Can you work these out from the model? Positions are in its coordinate system, mm. Face numbers are marked on the shaded views. A direction names the side the tool comes from. Round coordinates to 2 decimals unless told otherwise and drop trailing zeros. Order: outer loops, then holes, each group sorted by start corner. A loop starts at its lowest first (then second) coordinate and runs counter-clockwise, first axis right, second up. Notation, with made-up numbers: M 42.5,-29 L 87.5,-29 A28 cw 87.5,-9 Z; hole C 17,19.25 d9. An arc over 180 degrees is marked long. Answer as CSV lines item,"result". Start each with the question number.
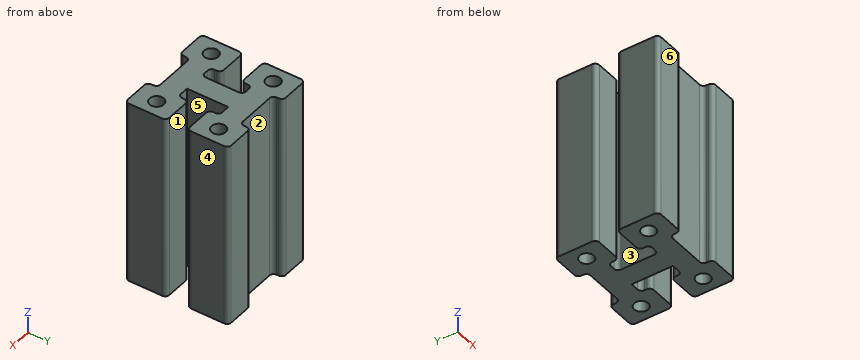
from build123d import *

# Parameters (mm, degrees)
SALIENTE_EXTRUIR1_DEPTH      = 22.4
REDONDEO1_R                  = 1
TALADRO_DE_MARGEN_PARA_M31_D = 3.4


with BuildPart() as part:
    # Croquis1 → Saliente-Extruir1 (new, symmetric)
    with BuildSketch(Plane(origin=(0, 0, 0), x_dir=(0, 1, 0), z_dir=(0, 0, 1))):
        Polygon((-5, 13), (5, 13), (5, 5.5), (2.5, 5.5), (2.5, 2.5), (12.5, 2.5), (12.5, 5.5), (10, 5.5), (10, 13), (20, 13), (20, 5.5), (17.5, 5.5), (17.5, -5.5), (20, -5.5), (20, -13), (10, -13), (10, -5.5), (12.5, -5.5), (12.5, -2.5), (2.5, -2.5), (2.5, -5.5), (5, -5.5), (5, -13), (-5, -13), (-5, -5.5), (-2.5, -5.5), (-2.5, 5.5), (-5, 5.5), align=None)
    extrude(amount=SALIENTE_EXTRUIR1_DEPTH, both=True)

    # Redondeo1
    redondeo1_edges = [part.edges().sort_by_distance(p)[0] for p in [
        (-5.5, -5, 0),
        (-13, -5, 0),
        (-13, 5, 0),
        (-5.5, 5, 0),
        (-5.5, 2.5, 0),
        (-2.5, 2.5, 0),
        (-2.5, 12.5, 0),
        (-5.5, 12.5, 0),
        (-5.5, 10, 0),
        (-13, 10, 0),
        (-13, 20, 0),
        (-5.5, 20, 0),
        (-5.5, 17.5, 0),
        (5.5, 17.5, 0),
        (5.5, 20, 0),
        (13, 20, 0),
        (13, 10, 0),
        (5.5, 10, 0),
        (5.5, 12.5, 0),
        (5.5, 2.5, 0),
        (5.5, 5, 0),
        (13, 5, 0),
        (13, -5, 0),
        (5.5, -5, 0),
        (5.5, -2.5, 0),
        (-5.5, -2.5, 0),
    ]]
    fillet(redondeo1_edges, radius=REDONDEO1_R)

    # Taladro de margen para M31 (through all)
    with Locations(Plane(origin=(0, 0, -22.4), x_dir=(1, 0, 0), z_dir=(0, 0, -1))):
        with Locations((-9.25, -15), (-9.25, 0), (9.25, 0), (9.25, -15)):
            Hole(TALADRO_DE_MARGEN_PARA_M31_D / 2)


solid = part.part
(1) I want a section at B-B on y = 0. Write out the boundary of the cut face in (x, z).
(2) I want a section at C-C on z = 1.5. Count the separate pieces of the cut face and the enclosed holes in it, and give its area (3 significant figures).
(3) I want a section at D-D on y = 15.75. Write out the boundary of the cut face in (x, z), and give its area (3 significant figures).
(4) I'm going to push flat-ended pins straight in: P1, Ø0.8, axis at x = -4, z = 1, coming from the +Y side; P2, Ø2, axis at x = 9.25, y = 15, coming from the -Z side; P3, Ø2, axis at x = 3.5, z = -8.5, coming from the -Y side; P4, Ø10, axis at x = 0, z = -6, coming from the -Y side. Where does each tip first touch, or does it pass through?
(5) If we mould it in two halves opening along X, with no side actions, what happens to the marked faces 4, 5 and 6? For each: +X half, -X half, draft (parallel to the pull), parting line (faces both ways), or undercut.
(6) I want a section at A-A on x = 9.25. Write out the boundary of the cut face in (y, z).
(7) For the marked faces 1, 2 and 3, which set-ups out of +Z, -Z, +X, -X, +Y, -Y let a thin tool reach every point of the face, with its end or its side?
(8) If I drill on line 1 along X through (y, z) = (15, 14); line 2 along Y through (x, z) = (-9.25, 12.5); line 3 along Y through (x, z) = (-11.25, 2), over which ranges is the centre line in solid material (lowest first)?
From the geometry:
1,outline,"M -13,-22.4 L -10.95,-22.4 L -10.95,22.4 L -13,22.4 Z; M -7.55,-22.4 L 7.55,-22.4 L 7.55,22.4 L -7.55,22.4 Z; M 10.95,-22.4 L 13,-22.4 L 13,22.4 L 10.95,22.4 Z"
2,separate pieces,"1"
2,enclosed holes,"4"
2,area,"422 mm²"
3,outline,"M -13,-22.4 L -10.78,-22.4 L -10.78,22.4 L -13,22.4 Z; M -7.72,-22.4 L 7.72,-22.4 L 7.72,22.4 L -7.72,22.4 Z; M 10.78,-22.4 L 13,-22.4 L 13,22.4 L 10.78,22.4 Z"
3,area,"891 mm²"
4,P1,"y = 17.5"
4,P2,"through"
4,P3,"y = -2.5"
4,P4,"y = -2.63"
5,face 4,"+X half"
5,face 5,"undercut"
5,face 6,"draft"
6,outline,"M -5,-22.4 L -1.7,-22.4 L -1.7,22.4 L -5,22.4 Z; M 1.7,-22.4 L 5,-22.4 L 5,22.4 L 1.7,22.4 Z; M 10,-22.4 L 13.3,-22.4 L 13.3,22.4 L 10,22.4 Z; M 16.7,-22.4 L 20,-22.4 L 20,22.4 L 16.7,22.4 Z"
7,face 1,"+Z, -Z, +X"
7,face 2,"+Z, -Z, +Y"
7,face 3,"+Z, -Z"
8,line 1,"-13 to -10.95, -7.55 to 7.55, 10.95 to 13"
8,line 2,"-5 to -1.7, 1.7 to 5, 10 to 13.3, 16.7 to 20"
8,line 3,"-5 to 5, 10 to 20"
